Verification items for this drawing (mm, ordinates from the low corner). A direction names the side the tool comes from. Give positions to 0.01 mm unless a question says otherwise; leave off trailing zeros. Order: outer loops, then holes, each group sorted by start corner. A loop starts at its lowest first (then second) coordinate and runs counter-clockwise, first axis right, second up.
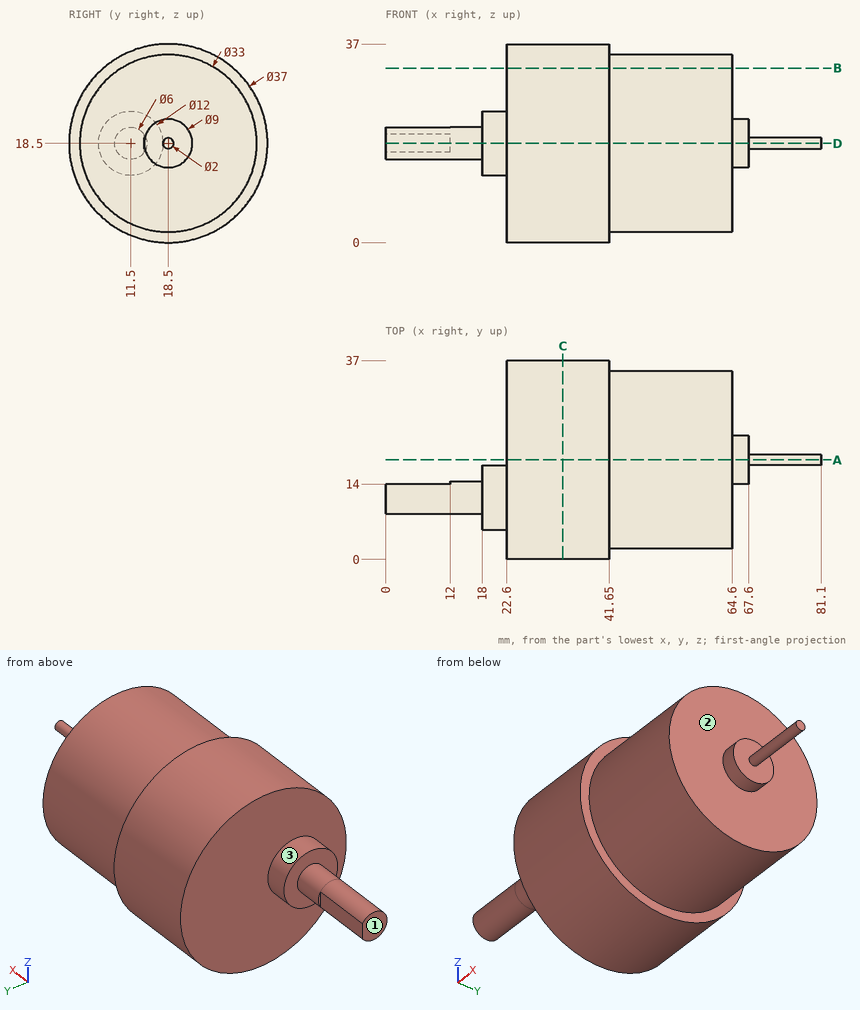
Q1. Cross-section at B-B, the plane z = 32.5. Record the boundary of the cut face in (x, y), and give its area (3 significant figures).
Q2. Access from +Z, -Z, +X, -X, +Y, -Y to the whole of each face (thin tool, end or side, straight path). Record for the marked faces 1, 2 and 3.
Q3. Cross-section at C-C, the plane x = 33. Record the boundary of the cut face in (y, z).
Q4. Gauge pin test, flat ends, axial feed: P1, Ø1, axis at x = 5.5, z = 19.5, coming from the +Y side; P2, Ø3, axis at x = 56, z = 31, coming from the -Y side; P3, Ø1.5, axis at y = 19.5, z = 11, coming from the -X side; P4, Ø4.5, axis at y = 17.5, z = 20, coming from the +X side. Record the tip position at first contact, or that the pin passes through.
Q5. Cross-section at D-D, the plane z = 18.5. Record the boundary of the cut face in (x, y).
Q6. Thickness scan on L1, parallel to X at y = 2.5, z = 12; L2, parallel to X at y = 28.5, z = 21; L3, parallel to Z at x = 62.5, y = 18. Record the ranges inside material, lowest first.
Q7. Cross-section at A-A, the plane y = 18.5. Record the boundary of the cut face in (x, z).
Answers follow:
1. outline: (22.6, 6.41) - (41.65, 6.41) - (41.65, 9.77) - (64.6, 9.77) - (64.6, 27.23) - (41.65, 27.23) - (41.65, 30.59) - (22.6, 30.59) - close
1. area: 862 mm2
2. face 1: +Z, -Z, -X, +Y, -Y
2. face 2: +X
2. face 3: -X
3. outline: circle Ø37 at (18.5, 18.5)
4. P1: stops at y = 14
4. P2: stops at y = 6.2
4. P3: stops at x = 22.6
4. P4: stops at x = 81.1
5. outline: (0, 8.5) - (18, 8.5) - (18, 5.5) - (22.6, 5.5) - (22.6, 0) - (41.65, 0) - (41.65, 2) - (64.6, 2) - (64.6, 14) - (67.6, 14) - (67.6, 17.5) - (81.1, 17.5) - (81.1, 19.5) - (67.6, 19.5) - (67.6, 23) - (64.6, 23) - (64.6, 35) - (41.65, 35) - (41.65, 37) - (22.6, 37) - (22.6, 17.5) - (18, 17.5) - (18, 14.5) - (12, 14.5) - (12, 14) - (0, 14) - close
6. L1: x = 22.6 to 41.65
6. L2: x = 22.6 to 64.6
6. L3: z = 2.01 to 34.99
7. outline: (22.6, 0) - (41.65, 0) - (41.65, 2) - (64.6, 2) - (64.6, 14) - (67.6, 14) - (67.6, 17.5) - (81.1, 17.5) - (81.1, 19.5) - (67.6, 19.5) - (67.6, 23) - (64.6, 23) - (64.6, 35) - (41.65, 35) - (41.65, 37) - (22.6, 37) - close
